from build123d import *

# Parameters (mm, degrees)
F1_DEPTH = 16
F2_W     = 9.0714404329
F2_H     = 45.9705627485
F2_W_2   = 9.9285595671
F3_DEPTH = 25
F5_DEPTH = 18.0322229203
F6_R     = 1.35
F7_DEPTH = 18.0322229203
F8_DEPTH = 18.0322229203


with BuildPart() as f1:
    # F0 (on Front) → F1 (new body)
    with BuildSketch(Plane.XZ):
        Polygon((0, 49), (0, 0), (1.5, 0), (1.5, 48.3786796564), (18.0312229203, 64.9099025767), (16.9705627485, 65.9705627485), align=None)
    extrude(amount=F1_DEPTH)

    # F2 (on Right) → F3 (cut)
    with BuildSketch(Plane.YZ):
        with Locations((2.0357202164, 42.9852813742)):
            Rectangle(F2_W, F2_H)
        with Locations((-18.4642797836, 42.9852813742)):
            Rectangle(F2_W_2, F2_H)
    extrude(amount=F3_DEPTH, mode=Mode.SUBTRACT)

    # F4 (on face) → F5 (cut, through all)
    with BuildSketch(Plane(origin=(0, 0, 0), x_dir=(0, -1, 0), z_dir=(-1, 0, 0))):
        with BuildLine():
            ThreePointArc((18, 10), (8, 0), (-2, 10))
            Line((-2, 10), (-2, -2.5))
            Line((-2, -2.5), (18, -2.5))
            Line((18, -2.5), (18, 10))
        make_face()
    extrude(amount=-F5_DEPTH, mode=Mode.SUBTRACT)

    # F6 (on face) → F7 (cut, through all)
    with BuildSketch(Plane(origin=(0, 0, 0), x_dir=(0, -1, 0), z_dir=(-1, 0, 0))):
        with Locations((13, 16)):
            Circle(F6_R)
        with Locations((3, 4)):
            Circle(F6_R)
    extrude(amount=-F7_DEPTH, mode=Mode.SUBTRACT)

    # F6 (on face) → F8 (cut, through all)
    with BuildSketch(Plane(origin=(0, 0, 0), x_dir=(0, -1, 0), z_dir=(-1, 0, 0))):
        with Locations((13, 16)):
            Circle(F6_R)
        with Locations((3, 4)):
            Circle(F6_R)
    extrude(amount=-F8_DEPTH, mode=Mode.SUBTRACT)


solid = f1.part
Can you work these out from the model? Positions are in its coordinate system, mm. A direction names the side the tool comes from. Give positions to 0.01 mm unless a question says otherwise; leave off trailing zeros. Loops run counter-clockwise (first coordinate to the right, second up) from the corner with the lowest first, then second, coordinate; pieces in that order, holes last. Notation, with made-up numbers: (-33, -24.5) - (17, -24.5) arc R22 ccw to (17, 2.5) - close; hole circle Ø1 at (33, 86). An arc over 180 degrees is marked (long way). Return JSON: item names as keys, results as strings.
1. I'm going to push flat-ended pins straight in: pin 1 Ø1.2 at (x, y) = (1, -1) entering from +Z; pin 2 Ø4 at (x, y) = (7.5, -6.5) entering from -Z; pin 3 Ø2 at (y, z) = (-7, 17) entering from +X. Where does each tip first touch, or does it pass through?
Output values:
{"pin 1": "stops at z = 20", "pin 2": "stops at z = 52.38", "pin 3": "stops at x = 1.5"}
2. If I drill on line 1 (Z direction, x = 0.5, y = -3); line 2 (X direction, y = -13, z = 18.5); line 3 (Z direction, x = 0.85, y = -13), over which ranges is the centre line in solid material (lowest first)?
Output values:
{"line 1": "z = 1.34 to 2.65, 5.35 to 49.5", "line 2": "x = 0 to 1.5", "line 3": "z = 1.34 to 14.65, 17.35 to 49.85"}
3. I want a section at A-A on z = 16. Please give me the cut outline in (x, y), and give its area (4 significant figures).
Output values:
{"outline": "(0, -16) - (1.5, -16) - (1.5, -14.35) - (0, -14.35) - close; (0, -11.65) - (1.5, -11.65) - (1.5, 0) - (0, 0) - close", "area": "19.95 mm²"}
4. For faces 5 (the face through (1, -13.5, 46)), 6 (the face through (1.5, -8, 24)), 7 (the face through (1, -1, 20)), which set-ups out of +Z, -Z, +X, -X, +Y, -Y let a thin tool reach every point of the face, with its end or its side?
Output values:
{"face 5": "+Z, +X, -X, -Y", "face 6": "-Z, +X, +Y, -Y", "face 7": "+Z, +X, -X, +Y"}
5. I want a section at D-D on x = 12.75. Please give me the cut outline in (y, z).
Output values:
{"outline": "(-13.5, 59.63) - (-2.5, 59.63) - (-2.5, 61.75) - (-13.5, 61.75) - close"}
6. I want a section at B-B on y = -3.25. Please give me the cut outline in (x, z).
Output values:
{"outline": "(0, 1.2) - (1.5, 1.2) - (1.5, 2.67) - (0, 2.67) - close; (0, 5.33) - (1.5, 5.33) - (1.5, 48.38) - (18.03, 64.91) - (16.97, 65.97) - (0, 49) - close"}
7. We'd pull the mould along Z, two halves only. Please class faces 1 (the face through (0.74, -3.62, 2.8)), 2 (the face through (1, -16, 12)), 3 (the face through (9.65, -7.92, 56.53)), 4 (the face through (0.74, -12.005, 16.912)): +Z half, -Z half, draft (parallel to the pull), parting line (faces both ways), or undercut.
Output values:
{"face 1": "undercut", "face 2": "draft", "face 3": "-Z half", "face 4": "undercut"}
8. I want a section at C-C on z = 31. Please give me the cut outline in (x, y), and give its area (3 significant figures).
Output values:
{"outline": "(0, -13.5) - (1.5, -13.5) - (1.5, -2.5) - (0, -2.5) - close", "area": "16.5 mm²"}
